```python
from build123d import *

# Parameters (mm, degrees)
F0_R     = 23.5
F0_R_2   = 22.5
F0_R_3   = 3
F1_DEPTH = 35
F2_START = 2
F0_R_4   = 2.75
F2_DEPTH = 31
F4_DEPTH = 6
F5_START = 23
F5_DEPTH = 12


# Not quite as in the source:
# - a fillet or chamfer that OpenCascade refuses, or shapes differently, is made with other operations: its cross-section is extruded or revolved along the edge and cut away or added


with BuildPart() as f1:
    # F0 (on Top) → F1 (new body)
    with BuildSketch(Plane.XY):
        Circle(F0_R)
        Circle(F0_R_2, mode=Mode.SUBTRACT)
        Circle(F0_R_2)
        with BuildLine():
            ThreePointArc((19.8808953521, 5), (20.3446351002, 2.5190916302), (20.5, 0))
            ThreePointArc((20.5, 0), (20.3446351002, -2.5190916302), (19.8808953521, -5))
            ThreePointArc((19.8808953521, -5), (14.4956890143, -14.4956890143), (5, -19.8808953521))
            ThreePointArc((5, -19.8808953521), (0, -20.5), (-5, -19.8808953521))
            ThreePointArc((-5, -19.8808953521), (-14.4956890143, -14.4956890143), (-19.8808953521, -5))
            ThreePointArc((-19.8808953521, -5), (-20.5, 0), (-19.8808953521, 5))
            ThreePointArc((-19.8808953521, 5), (-14.4956890143, 14.4956890143), (-5, 19.8808953521))
            ThreePointArc((-5, 19.8808953521), (0, 20.5), (5, 19.8808953521))
            ThreePointArc((5, 19.8808953521), (14.4956890143, 14.4956890143), (19.8808953521, 5))
        make_face(mode=Mode.SUBTRACT)
        with BuildLine():
            ThreePointArc((6, 0), (5.5432771953, 2.2961005937), (4.2426406878, 4.2426406864))
            ThreePointArc((4.2426406878, 4.2426406864), (7.8e-09, 6), (-4.2426406768, 4.2426406974))
            ThreePointArc((-4.2426406768, 4.2426406974), (-6, 7.9e-09), (-4.242640688, -4.2426406862))
            ThreePointArc((-4.242640688, -4.2426406862), (-1.21e-08, -6), (4.2426406709, -4.2426407033))
            ThreePointArc((4.2426406709, -4.2426407033), (5.5432771907, -2.2961006048), (6, 0))
        make_face()
        Polygon((-3.9, -2.2516660498), (-3.9, 2.2516660498), (0, 4.5033320997), (3.9, 2.2516660498), (3.9, -2.2516660498), (0, -4.5033320997), align=None, mode=Mode.SUBTRACT)
        with BuildLine():
            ThreePointArc((4.2426406878, 4.2426406864), (1.1585914251, 12.2294676794), (5, 19.8808953521))
            ThreePointArc((5, 19.8808953521), (0, 20.5), (-5, 19.8808953521))
            ThreePointArc((-5, 19.8808953521), (-1.1585914255, 12.2294676871), (-4.2426406768, 4.2426406974))
            ThreePointArc((-4.2426406768, 4.2426406974), (7.8e-09, 6), (4.2426406878, 4.2426406864))
        make_face()
        with BuildLine():
            ThreePointArc((19.8808953521, -5), (20.3446351002, -2.5190916302), (20.5, 0))
            ThreePointArc((20.5, 0), (20.3446351002, 2.5190916302), (19.8808953521, 5))
            ThreePointArc((19.8808953521, 5), (12.2294676803, 1.1585914252), (4.2426406878, 4.2426406864))
            ThreePointArc((4.2426406878, 4.2426406864), (5.5432771953, 2.2961005937), (6, 0))
            ThreePointArc((6, 0), (5.5432771907, -2.2961006048), (4.2426406709, -4.2426407033))
            ThreePointArc((4.2426406709, -4.2426407033), (12.2294676684, -1.1585914246), (19.8808953521, -5))
        make_face()
        with BuildLine():
            ThreePointArc((-5, -19.8808953521), (0, -20.5), (5, -19.8808953521))
            ThreePointArc((5, -19.8808953521), (1.1585914257, -12.2294676913), (4.2426406709, -4.2426407033))
            ThreePointArc((4.2426406709, -4.2426407033), (-1.21e-08, -6), (-4.242640688, -4.2426406862))
            ThreePointArc((-4.242640688, -4.2426406862), (-1.1585914251, -12.2294676792), (-5, -19.8808953521))
        make_face()
        with BuildLine():
            ThreePointArc((-4.242640688, -4.2426406862), (-6, 7.9e-09), (-4.2426406768, 4.2426406974))
            ThreePointArc((-4.2426406768, 4.2426406974), (-12.2294676726, 1.1585914248), (-19.8808953521, 5))
            ThreePointArc((-19.8808953521, 5), (-20.5, 0), (-19.8808953521, -5))
            ThreePointArc((-19.8808953521, -5), (-12.2294676805, -1.1585914252), (-4.242640688, -4.2426406862))
        make_face()
        Polygon((0, 4.5033320997), (-3.9, 2.2516660498), (-3.9, -2.2516660498), (0, -4.5033320997), (3.9, -2.2516660498), (3.9, 2.2516660498), align=None)
        Circle(F0_R_3, mode=Mode.SUBTRACT)
    extrude(amount=F1_DEPTH)

    # F0 (on Top) → F2 (join)
    with BuildSketch(Plane.XY.offset(F2_START)):
        Circle(F0_R_3)
        Circle(F0_R_4, mode=Mode.SUBTRACT)
    extrude(amount=F2_DEPTH)

    # F3: chamfer of 15 on 1 edges, made by hand


with BuildPart() as f3_tool2:
    # F3_s3 → F3_t4 (revolve)
    with BuildSketch(Plane.XZ):
        Polygon((18, 35), (3, 20), (3, 35), align=None)
    revolve(axis=Axis((0, 0, 35), (0, 0, 1)))

    split(bisect_by=Plane.XY.offset(33), keep=Keep.TOP)


with BuildPart() as f1_1:
    add(f1.part)

    # F3_t1: cut F3_tool2
    add(f3_tool2.part, mode=Mode.SUBTRACT)

    # F0 (on Top) → F4 (cut)
    with BuildSketch(Plane.XY):
        Polygon((0, 4.5033320997), (-3.9, 2.2516660498), (-3.9, -2.2516660498), (0, -4.5033320997), (3.9, -2.2516660498), (3.9, 2.2516660498), align=None)
        Circle(F0_R_3, mode=Mode.SUBTRACT)
    extrude(amount=F4_DEPTH, mode=Mode.SUBTRACT)

    # F0 (on Top) → F5 (cut)
    with BuildSketch(Plane.XY.offset(F5_START)):
        Polygon((0, 4.5033320997), (-3.9, 2.2516660498), (-3.9, -2.2516660498), (0, -4.5033320997), (3.9, -2.2516660498), (3.9, 2.2516660498), align=None)
        Circle(F0_R_3, mode=Mode.SUBTRACT)
    extrude(amount=F5_DEPTH, mode=Mode.SUBTRACT)


solid = f1_1.part
```
Design review of the part built by this model. Coordinates are the model's own, in mm. A direction names the side the tool comes from. Coordinates: 2 decimals unless noted, no trailing zeros. Write each loop counter-clockwise with the first axis right and the second up, starting at its lowest first coordinate (ties: lowest second). Pieces come first, ordered by that corner, then holes. Notation, with made-up numbers: M 82,-13 L 94,-13 A19 cw 94,7 Z; hole C -27.5,53 d4. An arc over 180 degrees is marked long. Answer as a JSON object with one key per item and string values.
Item 1: Machinability: for faces 1 (the cylindrical face through (-3, 0, 4)), 2 (the conical face through (0, 17, 34)), 3 (the cylindrical face through (14.6, -14.39, 17.26)), which of the approach directions +Z, -Z, +X, -X, +Y, -Y give a long, thin tool a straight path to every point of the face, cutting with its end or side? Answer none if there is none.
Outcome:
{"face 1": "-Z", "face 2": "+Z", "face 3": "+Z, -Z"}
Item 2: Add section A-A, the plane y = 0. Give the boundary of the cut face in (x, z).
Outcome:
{"outline": "M -23.5,0 L -3.9,0 L -3.9,6 L -3,6 L -3,2 L -2.75,2 L -2.75,33 L -3,33 L -3,23 L -3.9,23 L -3.9,33 L -16,33 L -18,35 L -23.5,35 Z; M 2.75,2 L 3,2 L 3,6 L 3.9,6 L 3.9,0 L 23.5,0 L 23.5,35 L 18,35 L 16,33 L 3.9,33 L 3.9,23 L 3,23 L 3,33 L 2.75,33 Z"}
Item 3: Insertion check: pin 1 Ø5 at (y, z) = (1, 29.5) entering from +X; pin 2 Ø7 at (x, y) = (0, 0) entering from -Z; pin 3 Ø12 at (x, z) = (2, 30) entering from -Y; pin 4 Ø2 at (x, z) = (-15, 19.5) entering from +Y. Each pin has a flat end and moves straight along its axis. Give the tip position at first contact, or say it passes through.
Outcome:
{"pin 1": "x = 23.5", "pin 2": "z = 2", "pin 3": "y = -23.5", "pin 4": "y = 18.87"}
Item 4: Add section C-C, the plane x = 12. Give the boundary of the cut face in (y, z).
Outcome:
{"outline": "M -20.21,0 L -16.62,0 L -16.62,35 L -20.21,35 Z; M -1.15,0 L 1.15,0 L 1.15,33 L -1.15,33 Z; M 16.62,0 L 20.21,0 L 20.21,35 L 16.62,35 Z"}
Item 5: Add section D-D, the plane y = 7. Give the boundary of the cut face in (x, z).
Outcome:
{"outline": "M -22.43,0 L -19.27,0 L -19.27,35 L -22.43,35 Z; M -2.26,0 L 2.26,0 L 2.26,33 L -2.26,33 Z; M 19.27,0 L 22.43,0 L 22.43,35 L 19.27,35 Z"}
Item 6: Add section B-B, the plane z = 26.5. Give the boundary of the cut face in (x, y), and give its area (3 significant figures).
Outcome:
{"outline": "C 0,0 d47; C 0,0 d6; hole M -19.88,-5 A20.5 ccw -5,-19.88 A10.57 ccw long Z; hole M -19.88,5 A10.57 ccw long -5,19.88 A20.5 ccw Z; hole M -3.9,-2.25 L 0,-4.5 L 3.9,-2.25 L 3.9,2.25 L 0,4.5 L -3.9,2.25 Z; hole C 0,0 d5.5; hole M 5,-19.88 A20.5 ccw 19.88,-5 A10.57 ccw long Z; hole M 5,19.88 A10.57 ccw long 19.88,5 A20.5 ccw Z", "area": "733 mm²"}
Item 7: Wall thickness on probe 1 along X at (y, z) = (10, 30); probe 2 along Y at (x, z) = (-17, 8.5); probe 3 along Y at (x, z) = (-6, 32.5): over which ranges is each line inside the solid? List them lowest first.
Outcome:
{"probe 1": "-21.27 to -17.9, -1.29 to 1.29, 17.9 to 21.27", "probe 2": "-16.22 to -11.46, -2.56 to 2.56, 11.46 to 16.22", "probe 3": "-22.72 to -19.6, -2.83 to 2.83, 19.6 to 22.72"}
